Autodesk Inventor part; units mm, degrees
ref_plane "YZ Plane" through (0, 0, 0) normal (1, 0, 0) x (0, 1, 0)
ref_plane "XZ Plane" through (0, 0, 0) normal (0, 1, 0) x (-1, 0, 0)
ref_plane "XY Plane" through (0, 0, 0) normal (0, 0, 1) x (1, 0, 0)
sketch "Sketch1" plane through (0, 0, 0) normal (0, 0, 1) x (1, 0, 0)
  circle A0 centre (0, 0) radius 35
  circle A1 centre (0, 0) radius 2.25
  dimension "d0" = 70
  dimension "d1" = 4.5
extrude "Extrusion1" add sketch "Sketch1" along normal blind 3
sketch "Sketch2" plane through (0, 0, 3) normal (0, 0, 1) x (1, 0, 0)
  circle A0 centre (0, 0) radius 32 construction
  point P0 (32, 0)
  dimension "d4" = 64
hole "Hole1" at (32, 0, 3) direction (0, 0, -1) diameter 3.4 end through all
pattern_circular "Circular Pattern1" count 4 over 360 about axis through (0, 0, 0) along (0, 0, 1) of "Hole1"
properties part number "plasma-box-anode-flange" material "Copper"
Work out the finished part from the listing and answer in its coordinate system (mm). Give positions to 0.01 mm unless a question says otherwise; leave off trailing zeros. Write each loop counter-clockwise with the first axis right and the second up, starting at its lowest first coordinate (ties: lowest second). Pieces come first, ordered by that corner, then holes.
Q1. Straight lines are drawn through the part: L1, parallel to Y at x = 0, z = 0.95; L2, parallel to Y at x = -31, z = 0.8; L3, parallel to Y at x = -28, z = 0.8. For each, find the intervals that lie inside material, in ascending order.
Answer:
L1: y = -35 to -33.7, -30.3 to -2.25, 2.25 to 30.3, 33.7 to 35
L2: y = -16.25 to -1.37, 1.37 to 16.25
L3: y = -21 to 21
Q2. The part is cut by section D-D on y = 32. Give the vertices of the cut face in (x, z).
Answer:
outline: (-14.18, 0) - (-1.7, 0) - (-1.7, 3) - (-14.18, 3) - close; (1.7, 0) - (14.18, 0) - (14.18, 3) - (1.7, 3) - close
Q3. The part is cut by section A-A on x = 0. Give the vertices of the cut face in (y, z).
Answer:
outline: (-35, 0) - (-33.7, 0) - (-33.7, 3) - (-35, 3) - close; (-30.3, 0) - (-2.25, 0) - (-2.25, 3) - (-30.3, 3) - close; (2.25, 0) - (30.3, 0) - (30.3, 3) - (2.25, 3) - close; (33.7, 0) - (35, 0) - (35, 3) - (33.7, 3) - close
Q4. Given pin 1 (1.5 mm diameter, centred on x = 2, z = 2.5, fed in from -Y), flat-ended and moving along its own axis, determine where the tip first touches the part or whether it passes through.
Answer:
pin 1: stops at y = -34.98
Q5. The part is cut by section C-C on z = 2.05. Give the vertices of the cut face in (x, y).
Answer:
outline: circle Ø70 at (0, 0); hole circle Ø3.4 at (-32, 0); hole circle Ø4.5 at (0, 0); hole circle Ø3.4 at (0, -32); hole circle Ø3.4 at (0, 32); hole circle Ø3.4 at (32, 0)
Q6. For a pull along X with two mould halves and no side action, classify faces 1 (the face through (-28, 21, 1)), 2 (the face through (-0.37, 33.66, 1.48)), 3 (the face through (0, -7, 3)) as released by +X, released by -X, zero draft, split by the parting line, or undercut.
Answer:
face 1: split by the parting line
face 2: undercut
face 3: zero draft
